The model under review builds one solid part; all positions refer to its coordinate system, in mm. Face numbers are marked on the shaded views. A direction names the side the tool comes from. Coordinates: 2 decimals unless noted, no trailing zeros. Write each loop counter-clockwise with the first axis right and the second up, starting at its lowest first coordinate (ties: lowest second). Pieces come first, ordered by that corner, then holes. Notation, with made-up numbers: M 73.25,68.25 L 114.25,68.25 A24 cw 114.25,100.25 Z; hole C -35.5,-11 d10. An arc over 180 degrees is marked long. Answer as CSV lines item,"result". Start each with the question number.
Autodesk Inventor part; units mm, degrees
ref_plane "YZ Plane" through (0, 0, 0) normal (1, 0, 0) x (0, 1, 0)
ref_plane "XZ Plane" through (0, 0, 0) normal (0, 1, 0) x (-1, 0, 0)
ref_plane "XY Plane" through (0, 0, 0) normal (0, 0, 1) x (1, 0, 0)
sketch "Sketch1" plane through (0, 0, 0) normal (0, 1, 0) x (-1, 0, 0)
  line L0 (-0.762, 12.7) -> (-0.762, 17.7225)
  line L1 (0.762, 12.7) -> (0.762, 17.7225)
  line L2 (-3.302, 12.7) -> (-3.302, 17.7225)
  line L3 (3.302, 12.7) -> (3.302, 17.7225)
  line L4 (3.302, 12.7) -> (3.302, 6.8674)
  line L5 (-3.302, 12.7) -> (-3.302, 6.8674)
  line L6 (-2.032, 18.9925) -> (-2.032, 18.9925)
  line L7 (2.032, 18.9925) -> (2.032, 18.9925)
  arc A0 (3.302, 17.7225) -> (2.032, 18.9925) centre (2.032, 17.7225) ccw
  arc A1 (2.032, 18.9925) -> (0.762, 17.7225) centre (2.032, 17.7225) ccw
  arc A2 (-0.762, 17.7225) -> (-2.032, 18.9925) centre (-2.032, 17.7225) ccw
  arc A3 (-2.032, 18.9925) -> (-3.302, 17.7225) centre (-2.032, 17.7225) ccw
  arc A4 (-0.762, 5.0225) -> (0.762, 5.0225) centre (0, 0) ccw
  line L8 (0.762, 12.7) -> (0.762, 5.0225)
  line L9 (-0.762, 12.7) -> (-0.762, 5.0225)
  arc A5 (-3.302, 6.8674) -> (-7.6187, -0.1405) centre (0, 0) ccw
  arc A6 (7.6187, -0.1405) -> (3.302, 6.8674) centre (0, 0) ccw
  line L10 (7.6187, -8.9561) -> (-7.6187, -8.9561)
  line L11 (7.6187, -8.9561) -> (7.6187, 0.1405)
  line L12 (-7.6187, -8.9561) -> (-7.6187, 0.1405)
  dimension "d3" = 2.54
  dimension "d4" = 2.54
  dimension "d5" = 1.27
  dimension "d6" = 10.16
  dimension "d7" = 1.524
  dimension "d8" = 1.524
  dimension "d9" = 12.7
  dimension "d10" = 12.7
extrude "Extrusion1" add sketch "Sketch1" along normal blind 25.4
sketch "Sketch3" plane through (3.302, 0, 17.7225) normal (1, 0, 0) x (0, 0, -1)
  line L0 (0, 25.4) -> (10.8551, 25.4)
  point P0 (17.7225, 0)
  point P1 (4.2489, 12.7)
  dimension "d24" = 12.7
hole "Hole2" at (3.302, 12.7, 13.4736) direction (-1, 0, 0) diameter 4.064 end through all
sketch "Sketch5" plane through (7.6187, 0, -8.9561) normal (0, 0, -1) x (-1, 0, 0)
  line L0 (2.5387, 0) -> (12.6987, 0)
  point P0 (7.6187, 0)
  point P1 (7.6187, 12.7)
  point P2 (8.3807, 0)
  point P3 (6.8567, 0)
  dimension "d34" = 12.7
hole "Hole3" at (0, 12.7, -8.9561) direction (0, 0, 1) diameter 3.556 depth 4.7625 tip angle 118
chamfer "Chamfer2" distance 2.286 angle 45 1 edges at (-0.0006, 10.922, -5.08)
sketch "Sketch6" plane through (7.6187, 0, -8.9561) normal (0, 0, -1) x (-1, 0, 0)
  circle A0 centre (7.6187, 12.7) radius 1.778
  line L0 (5.8407, 12.7) -> (9.3967, 12.7)
  line L1 (9.3967, 12.7) -> (9.3967, 25.4084)
  line L2 (9.3967, 25.4084) -> (5.8407, 25.4084)
  line L3 (5.8407, 25.4084) -> (5.8407, 12.7)
  point P0 (7.6187, 0)
extrude "Extrusion2" cut sketch "Sketch6" against normal blind 6.35 contours L0 A0 | A0 L3 L2 L1 picked at (8.0623, 13.093)
equation "\"d10\" = d9"
properties part number "pen holder 3" material "PBT Plastic"
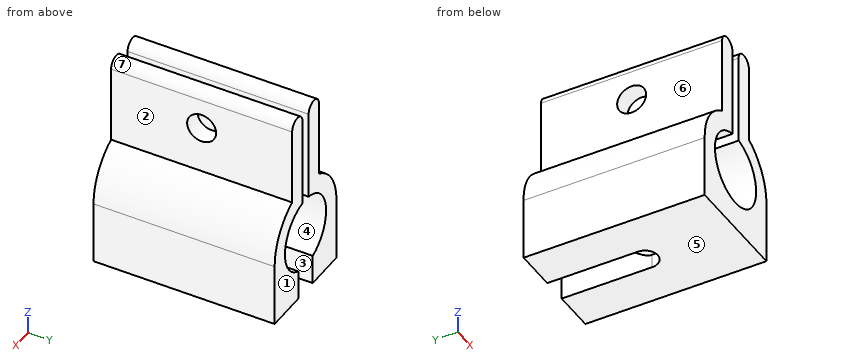
1) Take a section at C-C on z = 13.5. Give the boundary of the cut face in (x, y), and give its area (3 significant figures).
2) Tool access review of the marked faces 1, 2 and 3: name each direction out of +Z, -Z, +X, -X, +Y, -Y from which nothing blocks a thin tool from reaching the whole face with its end or side.
3) Clearance check with flat-ended pins moving along their axes: pin 1 Ø6.5 at (y, z) = (13.5, 8.5) entering from +X; pin 2 Ø4 at (y, z) = (22.5, 9) entering from -X; pin 3 Ø2.5 at (y, z) = (12.7, 13.47) entering from +X; pin 4 Ø3.5 at (y, z) = (7.5, 13) entering from +X. State where each tip first meets the part, or that it passes through.
4) Mouldability with a two-part tool opening along Z and no side actions: class the marked faces 4, 5, 6 and 7 as +Z half, -Z half, draft (parallel to the pull), parting line (faces both ways), or undercut.
5) Take a section at A-A on z = 9. Give the boundary of the cut face in (x, y).
6) To check wall thickness, follow line 1 (X direction, y = 13.75, z = 15.5); line 2 (X direction, y = 16.5, z = 0); line 3 (Z direction, x = -2.5, y = 12.7). State the ranges of each line that lie inside material, in increasing order. Write a range as [from, to].
7) Take a section at B-B on x = 4.75. Give the boundary of the cut face in (y, z).
Results:
1,outline,"M -3.3,0 L -0.76,0 L -0.76,10.67 L -3.3,10.67 Z; M -3.3,14.73 L -0.76,14.73 L -0.76,25.4 L -3.3,25.4 Z; M 0.76,0 L 3.3,0 L 3.3,10.67 L 0.76,10.67 Z; M 0.76,14.73 L 3.3,14.73 L 3.3,25.4 L 0.76,25.4 Z"
1,area,"108 mm²"
2,face 1,"+Z, -Z, +X, -X, +Y"
2,face 2,"+Z, +X, +Y, -Y"
2,face 3,"-Z, +Y"
3,pin 1,"stops at x = 5.52"
3,pin 2,"stops at x = -3.3"
3,pin 3,"passes through"
3,pin 4,"stops at x = 3.3"
4,face 4,"undercut"
4,face 5,"-Z half"
4,face 6,"draft"
4,face 7,"+Z half"
5,outline,"M -3.3,0 L -0.76,0 L -0.76,25.4 L -3.3,25.4 Z; M 0.76,0 L 3.3,0 L 3.3,25.4 L 0.76,25.4 Z"
6,line 1,"x = [-3.3, -0.76], [0.76, 3.3]"
6,line 2,"x = [-7.62, -5.08], [5.08, 7.62]"
6,line 3,"z = [-8.96, -5.7], [4.42, 11.44], [15.51, 18.9]"
7,outline,"M 0,-8.96 L 25.4,-8.96 L 25.4,-1.8 L 0,-1.8 Z; M 0,1.8 L 25.4,1.8 L 25.4,5.96 L 0,5.96 Z"
